The model under review builds one solid part; all positions refer to its coordinate system, in mm. A direction names the side the tool comes from. Coordinates: 2 decimals unless noted, no trailing zeros. Loops run counter-clockwise (first coordinate to the right, second up) from the corner with the lowest first, then second, coordinate; pieces in that order, holes last. Notation, with made-up numbers: M 13.25,54.25 L 69.25,54.25 A17 ccw 69.25,60.25 Z; hole C -20.75,6.25 d3. An arc over 180 degrees is marked long. Return JSON: item names as keys, results as strings.
Autodesk Inventor part; units mm, degrees
ref_plane "YZ Plane" through (0, 0, 0) normal (1, 0, 0) x (0, 1, 0)
ref_plane "XZ Plane" through (0, 0, 0) normal (0, 1, 0) x (-1, 0, 0)
ref_plane "XY Plane" through (0, 0, 0) normal (0, 0, 1) x (1, 0, 0)
sketch "Sketch1" plane through (0, 0, 0) normal (0, 1, 0) x (-1, 0, 0)
  line L0 (0, 0) -> (25.4, 0)
  line L1 (25.4, 0) -> (25.4, -50.8)
  line L2 (25.4, -50.8) -> (0, -50.8)
  line L3 (0, -50.8) -> (0, 0)
  dimension "d0" = 25.4
  dimension "d1" = 50.8
extrude "Extrusion1" add sketch "Sketch1" along normal blind 3.175
sketch "Sketch2" plane through (0, 3.175, 0) normal (0, 1, 0) x (1, 0, 0)
  line L0 (-25.4, 0) -> (0, 0)
  line L1 (0, 50.8) -> (-25.4, 50.8)
  line L2 (-25.4, 0) -> (-22.225, 0)
  line L3 (-22.225, 0) -> (-22.225, 50.8)
  line L4 (-22.225, 50.8) -> (-25.4, 50.8)
  line L5 (-25.4, 50.8) -> (-25.4, 0)
  line L6 (0, 0) -> (-3.175, 0)
  line L7 (-3.175, 0) -> (-3.175, 50.8)
  line L8 (-3.175, 50.8) -> (0, 50.8)
  line L9 (0, 50.8) -> (0, 0)
  dimension "d4" = 3.175
  dimension "d5" = 3.175
extrude "Extrusion2" add sketch "Sketch2" along normal blind 12.7 contours L5 L1 L3 L0 | L7 L1 L9 L0
sketch "Sketch3" plane through (-25.4, 0, -50.8) normal (-1, 0, 0) x (0, 0, 1)
  circle A0 centre (44.45, 7.62) radius 3.175
  line L0 (50.8, 0) -> (0, 0)
  line L1 (50.8, 0) -> (50.8, 15.875)
  dimension "d8" = 6.35
  dimension "d9" = 7.62
  dimension "d10" = 6.35
extrude "Extrusion3" cut sketch "Sketch3" against normal blind 25.4
properties part number "Manipulator2LeverAdapter"
1. Machinability: for faces 4 (the face through (-13, 3.175, -25)), 5 (the face through (-24, 15.875, -26)), which of the approach directions +Z, -Z, +X, -X, +Y, -Y give a long, thin tool a straight path to every point of the face, cutting with its end or side? Answer none if there is none.
Check values:
{"face 4": "+Z, -Z, +Y", "face 5": "+Z, -Z, +X, -X, +Y"}
2. Add section C-C on z = -14.5. Give the boundary of the cut face in (x, y) (3 decimals), plus the area to 3 significant figures.
Check values:
{"outline": "M -25.4,0 L 0,0 L 0,15.875 L -3.175,15.875 L -3.175,3.175 L -22.225,3.175 L -22.225,15.875 L -25.4,15.875 Z", "area": "161 mm²"}
3. Add section B-B on z = -6.35. Give the boundary of the cut face in (x, y) (3 decimals), plus the area to 3 significant figures.
Check values:
{"outline": "M -25.4,0 L 0,0 L 0,4.445 L -3.175,4.445 L -3.175,3.175 L -22.225,3.175 L -22.225,4.445 L -25.4,4.445 Z; M -25.4,10.795 L -22.225,10.795 L -22.225,15.875 L -25.4,15.875 Z; M -3.175,10.795 L 0,10.795 L 0,15.875 L -3.175,15.875 Z", "area": "121 mm²"}
4. Add section A-A on y = 7.62. Give the boundary of the cut face in (x, z) (3 decimals), plus the area to 3 significant figures.
Check values:
{"outline": "M -25.4,-50.8 L -22.225,-50.8 L -22.225,-9.525 L -25.4,-9.525 Z; M -25.4,-3.175 L -22.225,-3.175 L -22.225,0 L -25.4,0 Z; M -3.175,-50.8 L 0,-50.8 L 0,-9.525 L -3.175,-9.525 Z; M -3.175,-3.175 L 0,-3.175 L 0,0 L -3.175,0 Z", "area": "282 mm²"}
5. The part is to be moulded in two halves that separate along X. For faces 1 (the face through (-13, 0, -25)), 2 (the face through (0, 8, -26)), 3 (the face through (-22.225, 9, -25)), say which applies: released by +X, released by -X, zero draft, split by the parting line, or undercut.
Check values:
{"face 1": "zero draft", "face 2": "released by +X", "face 3": "undercut"}
6. To check wall thickness, follow line 1 (Y direction, x = -24.75, z = -6.35) (3 decimals); line 2 (X direction, y = 6, z = -22) (3 decimals); line 3 (Y direction, x = -12.5, z = -3.5) (3 decimals). State the ranges of each line that lie inside material, in increasing order.
Check values:
{"line 1": "0 to 4.445, 10.795 to 15.875", "line 2": "-25.4 to -22.225, -3.175 to 0", "line 3": "0 to 3.175"}
7. Add section D-D on x = -21. Give the boundary of the cut face in (y, z) (3 decimals), plus the area to 3 significant figures.
Check values:
{"outline": "M 0,-50.8 L 3.175,-50.8 L 3.175,0 L 0,0 Z", "area": "161 mm²"}
8. Insertion check: pin 1 Ø8.5 at (y, z) = (7.62, -6.35) entering from -X; pin 2 Ø9.5 at (x, z) = (-10, -28) entering from +Y (3 decimals). Each pin has a flat end and moves straight along its axis. Give the tip position at first contact, or say it passes through.
Check values:
{"pin 1": "x = -25.4", "pin 2": "y = 3.175"}
